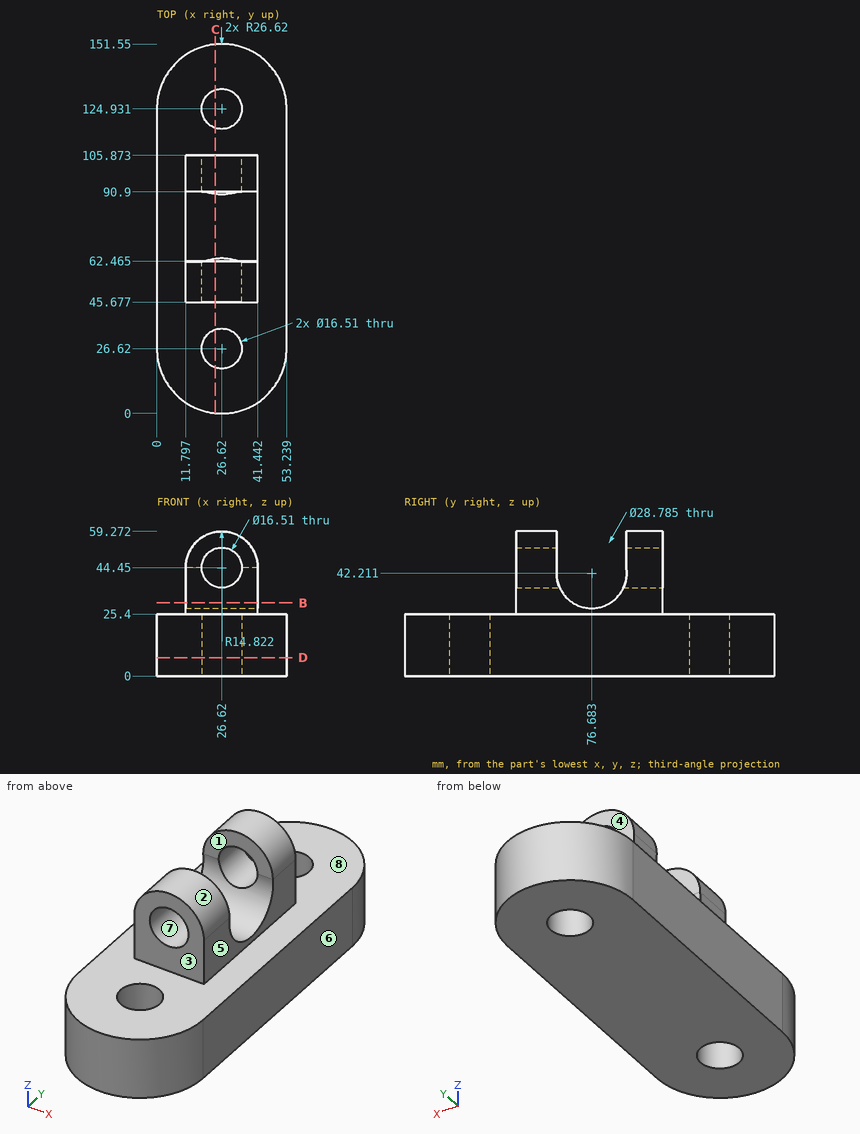
The drawing under review shows one solid part. Ordinate dimensions are in mm from its lowest x, y, z. A direction names the side the tool comes from. Give positions to 0.01 mm unless a question says otherwise; leave off trailing zeros. Order: outer loops, then holes, each group sorted by start corner. A loop starts at its lowest first (then second) coordinate and runs counter-clockwise, first axis right, second up. Notation, with made-up numbers: M -0.75,75 L 58.25,75 A24 cw 58.25,94 Z; hole C 85.5,8.5 d9. An arc over 180 degrees is marked long. Answer in a Markdown table with one row per item. Add a question column.
1. Add section C-C on x = 24. State the section outline as (y, z) points (1 decimal).
2. Mouldability with a two-part tool opening along Z and no side actions: class the marked faces 6, 7 and 8 as released by +Z, released by -Z, zero draft, split by the parting line, or undercut.
3. To check wall thickness, follow line 1 along Y through (x, z) = (40, 47) (1 decimal); line 2 along Z through (x, y) = (18, 37.5); line 3 along Y through (x, z) = (13, 39). State the ranges of each line that lie inside material, in increasing order.
4. Add section D-D on z = 7.5. State the section outline as (x, y) points (1 decimal), plus the area to 3 significant figures.
5. For pin 1 Ø7.5 at (x, z) = (32, 51) entering from +Y; pin 2 Ø3 at (y, z) = (20.5, 14) entering from -X; pin 3 Ø21.5 at (x, z) = (26.62, 44.45) entering from -Y; pin 4 Ø15 at (x, z) = (26.62, 44.45) entering from +Y, all flat-tipped, find the tip position at first contact; note any pin that passes through.
6. Machinability: for the marked faces 1, 2, 3, 4 and 5, which of the approach directions +Z, -Z, +X, -X, +Y, -Y give a long, thin tool a straight path to every point of the face, cutting with its end or side? Answer none if there is none.
7. Add section B-B on z = 30. State the section outline as (x, y) points.
The answers:
| question | item | result |
|---|---|---|
| 1 | outline | M 0.1,0 L 18.8,0 L 18.8,25.4 L 0.1,25.4 Z; M 34.4,0 L 117.1,0 L 117.1,25.4 L 105.9,25.4 L 105.9,36.6 L 89.9,36.6 A14.4 cw 63.4,36.6 L 45.7,36.6 L 45.7,25.4 L 34.4,25.4 Z; M 45.7,52.3 L 62.5,52.3 L 62.5,59 L 45.7,59 Z; M 90.9,52.3 L 105.9,52.3 L 105.9,59 L 90.9,59 Z; M 132.8,0 L 151.4,0 L 151.4,25.4 L 132.8,25.4 Z |
| 2 | face 6 | zero draft |
| 2 | face 7 | undercut |
| 2 | face 8 | released by +Z |
| 3 | line 1 | 45.7 to 62.5, 90.9 to 105.9 |
| 3 | line 2 | 0 to 25.4 |
| 3 | line 3 | 45.68 to 62.65, 90.71 to 105.87 |
| 4 | outline | M 0,26.6 A26.6 ccw 53.2,26.6 L 53.2,124.9 A26.6 ccw 0,124.9 Z; hole C 26.6,26.6 d16.5; hole C 26.6,124.9 d16.5 |
| 4 | area | 7,030 mm2 |
| 5 | pin 1 | y = 105.87 |
| 5 | pin 2 | x = 0.4 |
| 5 | pin 3 | y = 45.68 |
| 5 | pin 4 | through |
| 6 | face 1 | +Z, +X, -X |
| 6 | face 2 | +Z, +Y, -Y |
| 6 | face 3 | +Z, +X, -X, -Y |
| 6 | face 4 | +Z, +X, -X, +Y |
| 6 | face 5 | +Z, +X, +Y, -Y |
| 7 | outline | M 11.8,45.68 L 41.44,45.68 L 41.44,69.06 L 11.8,69.06 Z; M 11.8,84.3 L 41.44,84.3 L 41.44,105.87 L 11.8,105.87 Z |
